Here's how the part is built. I have some questions about the finished solid (model axes, mm). Coordinates: 2 decimals unless noted, no trailing zeros. Loops run counter-clockwise (first coordinate to the right, second up) from the corner with the lowest first, then second, coordinate; pieces in that order, holes last. Notation, with made-up numbers: M 75,-23 L 91,-23 A27 cw 91,6 Z; hole C 80.5,50 d8. An arc over 180 degrees is marked long. Use one line per item in the form item = value. Start each with the question number.
(1) Imagine slicing it at A-A, the plane z = 20. Please give me the cut outline in (x, y), and give its area (3 significant figures).
(2) Imagine slicing it at C-C, the plane x = 0.55. State how many separate pieces and enclosed holes the cut face has, and give its area (3 significant figures).
(3) Will these pins go through, and if not, where does the flat tip stop? P1, Ø3.5, axis at y = -8.37, z = -1.48, coming from the -X side; P2, Ø1.9, axis at y = -26.8, z = 13, coming from the +X side; P3, Ø0.6, axis at x = 0.5, z = 23, coming from the +Y side.
(4) Imagine slicing it at D-D, the plane z = -3.5. Please give me the cut outline in (x, y), and give its area (3 significant figures).
(5) Imagine slicing it at B-B, the plane y = -11.5. Please give me the cut outline in (x, z), and give its area (3 significant figures).
(6) Please list where these lines run through material, in increasing order: L1, parallel to Z at x = 1.95, y = -8; L2, parallel to Y at x = 0.3, z = 28; L3, parallel to Z at x = 0.5, y = -27.
Autodesk Inventor part; units mm, degrees
ref_plane "YZ Plane" through (0, 0, 0) normal (1, 0, 0) x (0, 1, 0)
ref_plane "XZ Plane" through (0, 0, 0) normal (0, 1, 0) x (-1, 0, 0)
ref_plane "XY Plane" through (0, 0, 0) normal (0, 0, 1) x (1, 0, 0)
sketch "スケッチ1" plane through (0, 0, 0) normal (1, 0, 0) x (0, 1, 0)
  line L0 (-29.3, 41) -> (-29.3, 9)
  line L1 (-29.3, 25) -> (-24.3, 25) construction
  line L2 (-26.8, 31) -> (-24.3, 31) construction
  line L3 (-24.3, 31) -> (-24.3, 19) construction
  line L4 (-24.3, 19) -> (-26.8, 19) construction
  line L5 (-26.8, 19) -> (-26.8, 31) construction
  line L6 (-26.8, 31) -> (-24.3, 19) construction
  line L7 (-24.3, 31) -> (-26.8, 19) construction
  circle A0 centre (-26.8, 37) radius 1.6
  line L8 (-26.8, 70.0011) -> (-26.8, -20.0011) construction
  line L9 (-29.3, 41) -> (-24.3, 41)
  circle A1 centre (0, 0) radius 5.05
  line L10 (-1.476, 8.3709) -> (1.476, -8.3709) construction
  circle A2 centre (-1.476, 8.3709) radius 1.35
  arc A3 (-7.6162, -7.6162) -> (10.7709, 0) centre (0, 0) ccw
  line L11 (-26.85, 31.05) -> (-24.25, 31.05)
  line L12 (-24.25, 31.05) -> (-24.25, 18.95)
  line L13 (-24.25, 18.95) -> (-26.85, 18.95)
  line L14 (-26.85, 18.95) -> (-26.85, 31.05)
  line L15 (-26.85, 31.05) -> (-24.25, 18.95) construction
  line L16 (-24.25, 31.05) -> (-26.85, 18.95) construction
  arc A4 (-24.25, 28.95) -> (-24.25, 31.05) centre (-24.25, 30) ccw
  line L17 (-25.55, 31) -> (-25.55, 19) construction
  arc A5 (-26.85, 31.05) -> (-26.85, 28.95) centre (-26.85, 30) ccw
  arc A6 (-24.25, 18.95) -> (-24.25, 21.05) centre (-24.25, 20) ccw
  arc A7 (-26.85, 21.05) -> (-26.85, 18.95) centre (-26.85, 20) ccw
  circle A8 centre (-26.8, 13) radius 1.6
  line L18 (-14.1813, 36.8087) -> (10.7709, 11.8566)
  line L19 (10.7709, 11.8566) -> (10.7709, 0)
  line L20 (-20.6489, 5.4166) -> (-7.6162, -7.6162)
  circle A9 centre (-6.9628, 4.8754) radius 1.35
  circle A10 centre (-8.3709, -1.476) radius 1.35
  circle A11 centre (0, 0) radius 16 construction
  arc A12 (-14.1813, 36.8087) -> (-24.3, 41) centre (-24.3, 26.6899) ccw
  line L21 (-20.3, 36.1924) -> (-20.3, 10.2769)
  arc A13 (-17.0097, 33.9803) -> (-20.3, 36.1924) centre (-24.3, 26.6899) ccw
  line L22 (6.7709, 10.0706) -> (6.7709, 8.438)
  circle A14 centre (-1.476, 8.3709) radius 2.4 construction
  line L23 (1.002, 15.9686) -> (-17.0097, 33.9803)
  arc A15 (-20.6489, 5.4166) -> (-29.3, 9) centre (-29.3, -3.2345) ccw
  circle A16 centre (-4.8754, -6.9628) radius 1.35
  circle A17 centre (1.476, -8.3709) radius 1.35
  arc A18 (-17.8205, 8.245) -> (-20.3, 10.2769) centre (-29.3, -3.2345) ccw
  line L24 (-1.093, -4.9303) -> (8.1951, -6.9894)
  line L25 (1.093, 4.9303) -> (10.7709, 2.7848)
  circle A19 centre (6.9628, -4.8754) radius 1.35
  circle A20 centre (8.3709, 1.476) radius 1.35
  circle A21 centre (4.8754, 6.9628) radius 1.35
  circle A22 centre (-6.9628, 4.8754) radius 2.4 construction
  circle A23 centre (-8.3709, -1.476) radius 2.4 construction
  circle A24 centre (-4.8754, -6.9628) radius 2.4 construction
  circle A25 centre (1.476, -8.3709) radius 2.4 construction
  circle A26 centre (6.9628, -4.8754) radius 2.4 construction
  circle A27 centre (8.3709, 1.476) radius 2.4 construction
  circle A28 centre (4.8754, 6.9628) radius 2.4 construction
  line L26 (6.9628, -4.8754) -> (8.3709, 1.476) construction
  line L27 (-17.8205, 8.245) -> (-15.0385, 5.463)
  arc A29 (1.002, 15.9686) -> (-15.0385, 5.463) centre (0, 0) ccw
  point P0 (-25.55, 25)
  point P1 (-26.8, 25)
  point P2 (-24.25, 21.05)
  point P3 (-26.85, 21.05)
  point P4 (-26.85, 28.95)
  point P5 (-0.8769, 4.9733)
  point P6 (0.8769, -4.9733)
  dimension "d0" = 5
  dimension "d1" = 32
  dimension "d2" = 2.5
  dimension "d3" = 12
  dimension "d4" = 3.2
  dimension "d5" = 5
  dimension "d6" = 10.1
  dimension "d7" = 17
  dimension "d8" = 2.7
  dimension "d10" = 29.3
  dimension "d11" = 1.05
  dimension "d12" = 0.05
  dimension "d13" = 0.05
  dimension "d14" = 24
  dimension "d15" = 25
  dimension "d19" = 360
  dimension "d23" = 32
  dimension "d24" = 45
  dimension "d31" = 4
  dimension "d32" = 4
  dimension "d37" = 4.8
  dimension "d46" = 4
  dimension "d47" = 4
  dimension "d53" = 360
  dimension "d56" = 10
extrude "押し出し1" add sketch "スケッチ1" along normal blind 2 contours L9 A12 L18 L19 L25 A1 L24 A3 L20 A15 L0 | A9 | A16
fillet "フィレット1" radius 2 4 edges at (1, -20.3, 36.1924) (1, -20.3, 10.2769) (1, -15.0385, 5.463) (1, 1.002, 15.9686)
fillet "フィレット2" radius 2 3 edges at (1, 10.7709, 11.8566) (1, 8.1951, -6.9894) (1, 10.7709, 2.7848)
equation "\"d13\" = d12"
properties part number "Shoulder_side_frame" material "アルミニウム 2014-T4"
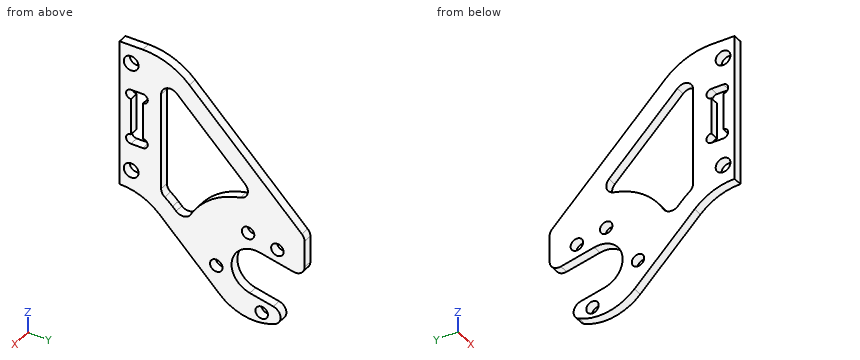
Answer:
q1.outline = M 0,-29.3 L 2,-29.3 L 2,-27.9 L 0,-27.9 Z; M 0,-23.2 L 2,-23.2 L 2,-20.3 L 0,-20.3 Z; M 0,-3.03 L 2,-3.03 L 2,2.63 L 0,2.63 Z
q1.area = 19.9 mm²
q2.separate_pieces = 1
q2.enclosed_holes = 8
q2.area = 796 mm²
q3.P1 = 0
q3.P2 = through
q3.P3 = -0.07
q4.outline = M 0,-11.73 L 2,-11.73 L 2,-3.64 L 0,-3.64 Z
q4.area = 16.2 mm²
q5.outline = M 0,-3.73 L 2,-3.73 L 2,11.12 L 0,11.12 Z; M 0,28.47 L 2,28.47 L 2,34.13 L 0,34.13 Z
q5.area = 41.0 mm²
q6.L1 = -7.23 to -2.77, -0.18 to 13.86, 24.97 to 30.63
q6.L2 = -29.3 to -26.85, -24.25 to -20.3, -11.03 to -5.37
q6.L3 = 8.78 to 11.41, 14.59 to 18.96, 21.04 to 28.96, 31.04 to 35.41, 38.59 to 41
